Source: CAD feature listing. Evaluate the final solid. Frame: model axes, mm. Round coordinates to 2 decimals unless told otherwise and drop trailing zeros. Order: outer loops, then holes, each group sorted by start corner. A loop starts at its lowest first (then second) coordinate and runs counter-clockwise, first axis right, second up. Notation, with made-up numbers: M 14,-6.5 L 25,-6.5 A27 ccw 25,26.5 Z; hole C 23,34 d5. An arc over 180 degrees is marked long. Use one line per item in the form item = value. Start each with the question number.
Q1. Material intervals for probe 1 along Z at (x, y) = (40, 2.25); probe 2 along Z at (x, y) = (68, 1.35), sorted ascending.
Q2. Section B-B (x = 55). Return the cut outline in (y, z).
Q3. Section A-A (z = -5). Return the cut outline in (x, y).
Q4. Section C-C (y = 1.75). Return the cut outline in (x, z).
Q5. Contact query for a flat-ended pin moving along its axis: pin 1 (2 mm diameter, centred on x = 63.5, y = 2, fed in from +Z). Output: stop coordinate, or through.
Q6. Section D-D (x = 11). Return the cut outline in (y, z), plus the area to 3 significant figures.
Q7. Pull-direction query (X, two-part tool) for faces 1 (the cylindrical face through (55.751, 1.726, -2.615)), 2 (the flat face through (47, 0, -5)), 3 (the flat face through (95, 2, -5)); classes: pulls with the +X half, pulls with the -X half, needs draft (parallel to the pull), parting line crosses it, or undercut.
from build123d import *

# Parameters (mm, degrees)
SKETCH1_W           = 150
SKETCH1_H           = 10
SKETCH1_R           = 2.5
BOSS_EXTRUDE1_DEPTH = 6
SKETCH2_W           = 10
SKETCH2_H           = 6
CUT_EXTRUDE1_DEPTH  = 55
SKETCH3_W           = 95
SKETCH3_H           = 10
CUT_EXTRUDE2_DEPTH  = 2.5


with BuildPart() as part:
    # Sketch1 → Boss-Extrude1 (new body)
    with BuildSketch(Plane(origin=(0, 0, 0), x_dir=(1, 0, 0), z_dir=(0, 1, 0))):
        with Locations((75, 5)):
            Rectangle(SKETCH1_W, SKETCH1_H)
        with Locations(Location((145, 5, 0), (0, 0, 270))):
            Circle(SKETCH1_R, mode=Mode.SUBTRACT)
        with Locations(Location((130, 5, 0), (0, 0, 270))):
            Circle(SKETCH1_R, mode=Mode.SUBTRACT)
        with Locations(Location((115, 5, 0), (0, 0, 270))):
            Circle(SKETCH1_R, mode=Mode.SUBTRACT)
        with Locations(Location((100, 5, 0), (0, 0, 270))):
            Circle(SKETCH1_R, mode=Mode.SUBTRACT)
        with Locations(Location((85, 5, 0), (0, 0, 270))):
            Circle(SKETCH1_R, mode=Mode.SUBTRACT)
        with Locations(Location((70, 5, 0), (0, 0, 270))):
            Circle(SKETCH1_R, mode=Mode.SUBTRACT)
        with Locations(Location((55, 5, 0), (0, 0, 270))):
            Circle(SKETCH1_R, mode=Mode.SUBTRACT)
        with Locations(Location((40, 5, 0), (0, 0, 270))):
            Circle(SKETCH1_R, mode=Mode.SUBTRACT)
        with Locations(Location((25, 5, 0), (0, 0, 270))):
            Circle(SKETCH1_R, mode=Mode.SUBTRACT)
        with Locations(Location((10, 5, 0), (0, 0, 270))):
            Circle(SKETCH1_R, mode=Mode.SUBTRACT)
    extrude(amount=BOSS_EXTRUDE1_DEPTH)

    # Sketch2 → Cut-Extrude1 (cut)
    with BuildSketch(Plane(origin=(150, 0, 0), x_dir=(0, 0, -1), z_dir=(1, 0, 0))):
        with Locations((5, 3)):
            Rectangle(SKETCH2_W, SKETCH2_H)
    extrude(amount=-CUT_EXTRUDE1_DEPTH, mode=Mode.SUBTRACT)

    # Sketch3 → Cut-Extrude2 (cut)
    with BuildSketch(Plane(origin=(0, 6, 0), x_dir=(1, 0, 0), z_dir=(0, 1, 0))):
        with Locations((47.5, 5)):
            Rectangle(SKETCH3_W, SKETCH3_H)
    extrude(amount=-CUT_EXTRUDE2_DEPTH, mode=Mode.SUBTRACT)


solid = part.part
Results list:
q1.probe_1 = -10 to -7.5, -2.5 to 0
q1.probe_2 = -10 to -6.5, -3.5 to 0
q2.outline = M 0,-10 L 3.5,-10 L 3.5,-7.5 L 0,-7.5 Z; M 0,-2.5 L 3.5,-2.5 L 3.5,0 L 0,0 Z
q3.outline = M 0,0 L 7.5,0 L 7.5,3.5 L 0,3.5 Z; M 12.5,0 L 22.5,0 L 22.5,3.5 L 12.5,3.5 Z; M 27.5,0 L 37.5,0 L 37.5,3.5 L 27.5,3.5 Z; M 42.5,0 L 52.5,0 L 52.5,3.5 L 42.5,3.5 Z; M 57.5,0 L 67.5,0 L 67.5,3.5 L 57.5,3.5 Z; M 72.5,0 L 82.5,0 L 82.5,3.5 L 72.5,3.5 Z; M 87.5,0 L 95,0 L 95,3.5 L 87.5,3.5 Z
q4.outline = M 0,-10 L 95,-10 L 95,0 L 0,0 Z; hole C 10,-5 d5; hole C 25,-5 d5; hole C 40,-5 d5; hole C 55,-5 d5; hole C 70,-5 d5; hole C 85,-5 d5
q5.pin_1 = 0
q6.outline = M 0,-10 L 3.5,-10 L 3.5,-7.29 L 0,-7.29 Z; M 0,-2.71 L 3.5,-2.71 L 3.5,0 L 0,0 Z
q6.area = 19.0 mm2
q7.face_1 = undercut
q7.face_2 = needs draft
q7.face_3 = pulls with the +X half
